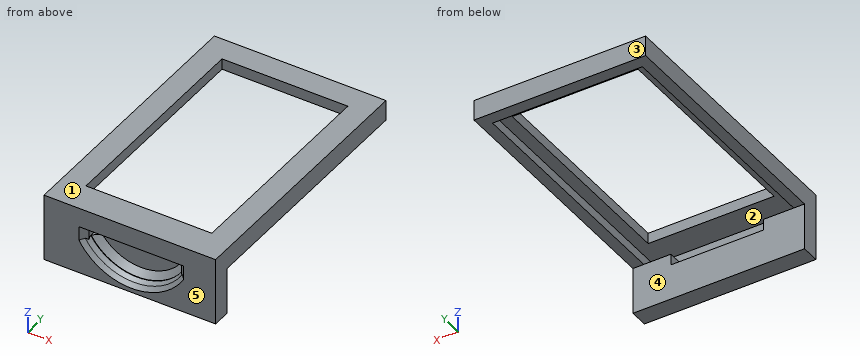
Autodesk Fusion 360 part; units mm, degrees
sketch "Sketch1" plane through (0, 0, 0) normal (0, 0, 1) x (1, 0, 0)
  line L0 (0, 0) -> (24.5, 0)
  line L1 (24.5, 0) -> (24.5, 42)
  line L2 (24.5, 42) -> (0, 42)
  line L3 (0, 42) -> (0, 0)
  line L4 (5, 39.4) -> (20, 39.4)
  line L5 (20, 39.4) -> (20, 24.4)
  line L6 (20, 24.4) -> (5, 24.4)
  line L7 (5, 24.4) -> (5, 39.4)
  dimension "d1" = 24.5
  dimension "d2" = 42
  dimension "d3" = 15
  dimension "d4" = 15
  dimension "d5" = 5
  dimension "d6" = 2.6
extrude "Extrude1" add sketch "Sketch1" along normal blind 1.2 contours L0 L1 L2 L3 | L4 L5 L6 L7 makes body 1
extrude "Extrude2" add sketch "Sketch1" against normal blind 1.85 contours L4 L5 L6 L7 bodies 1
sketch "Sketch2" plane through (0, 42, 0) normal (0, 1, 0) x (-1, 0, 0)
  line L0 (-24.5, 0) -> (0, 0)
  line L1 (0, 0) -> (0, 1.2)
  line L2 (0, 1.2) -> (-24.5, 1.2)
  line L3 (-24.5, 1.2) -> (-24.5, 0)
  line L4 (-26.5, 3.2) -> (2, 3.2)
  line L5 (2, 3.2) -> (2, -8)
  line L6 (2, -8) -> (-26.5, -8)
  line L7 (-26.5, -8) -> (-26.5, 3.2)
  line L8 (-20, 0) -> (-5, 0)
  line L9 (-5, 0) -> (-5, -1.85)
  line L10 (-5, -1.85) -> (-20, -1.85)
  line L11 (-20, -1.85) -> (-20, 0)
  line L12 (-20.2, 0.2) -> (-4.8, 0.2)
  line L13 (-4.8, 0.2) -> (-4.8, -2.05)
  line L14 (-4.8, -2.05) -> (-20.2, -2.05)
  line L15 (-20.2, -2.05) -> (-20.2, 0.2)
  line L16 (-24.7, 1.4) -> (0.2, 1.4)
  line L17 (0.2, 1.4) -> (0.2, -0.2)
  line L18 (0.2, -0.2) -> (-24.7, -0.2)
  line L19 (-24.7, -0.2) -> (-24.7, 1.4)
  arc A0 (-20.2, -2.05) -> (-4.8, -2.05) centre (-12.5, 2.7935) ccw
  line L20 (-26.5, 1.4) -> (2, 1.4)
  line L21 (2, 1.4) -> (2, 3.2)
  line L22 (2, 3.2) -> (-26.5, 3.2)
  line L23 (-26.5, 3.2) -> (-26.5, 1.4)
  line L24 (0.2, -0.2) -> (2, -0.2)
  line L25 (2, -0.2) -> (2, 1.4)
  line L26 (2, 1.4) -> (0.2, 1.4)
  line L27 (0.2, 1.4) -> (0.2, -0.2)
  line L28 (-24.7, -0.2) -> (-26.5, -0.2)
  line L29 (-26.5, -0.2) -> (-26.5, 1.4)
  line L30 (-26.5, 1.4) -> (-24.7, 1.4)
  line L31 (-24.7, 1.4) -> (-24.7, -0.2)
  dimension "d11" = 2
  dimension "d12" = 8
  dimension "d13" = 2
  dimension "d14" = 2
  dimension "d15" = 0.2
  dimension "d16" = 0.2
  dimension "d17" = 0.2
  dimension "d18" = 0.2
  dimension "d19" = 0.2
  dimension "d20" = 0.2
  dimension "d21" = 0.2
  dimension "d22" = 0.2
  dimension "d27" = 9.0967
  dimension "d33" = 0.2
extrude "Extrude3" add sketch "Sketch2" along normal blind 3 separate body contours L5 L6 L7 L13 L15 L18 A0 L24 L28 | L14 A0 | L7 L19 L20 L28 L29 L30 L31 | L5 L17 L20 L24 L25 L26 L27 | L4 L5 L7 L16 L20 L21 L22 L23 L26 L30 makes body 2
extrude "Extrude4" add sketch "Sketch2" along normal blind 0.4 contours L0 L8 L12 L13 L15 | L0 L1 L2 L3 L13 L15 L16 L17 L18 L19 L20 L27 L31 | L0 L1 L2 L3 L12 L13 L15 bodies 2
extrude "Extrude5" cut sketch "Sketch2" along normal blind 2.6 contours L14 A0 bodies 2
chamfer "Chamfer1" distance 1 angle 45 1 edges at (12.5, 44.6, -6.3032) on bodies 2
chamfer "Chamfer2" distance 1 angle 45 3 edges at (12.5, 42, -6.3032) (20.2, 42, -1.025) (4.8, 42, -1.025) on bodies 2
chamfer "Chamfer3" distance 0.5 angle 45 1 edges at (12.5, 43, -6.3032) on bodies 2
extrude "Extrude6" add sketch "Sketch2" along normal blind 44.6 contours L7 L19 L20 L28 L29 L30 L31 | L5 L17 L20 L24 L25 L26 L27 | L4 L5 L7 L16 L20 L21 L22 L23 L26 L30 bodies 2
sketch "Sketch3" plane through (0, 0, 1.4) normal (0, 0, -1) x (1, 0, 0)
  line L0 (24.7, -42.4) -> (-0.2, -42.4)
  line L1 (-0.2, -42.4) -> (-0.2, -86.6)
  line L2 (-0.2, -86.6) -> (24.7, -86.6)
  line L3 (24.7, -86.6) -> (24.7, -42.4)
  line L4 (-0.2, -86.6) -> (24.7, -86.6)
  line L5 (24.7, -86.6) -> (24.7, -84.6)
  line L6 (24.7, -84.6) -> (-0.2, -84.6)
  line L7 (-0.2, -84.6) -> (-0.2, -86.6)
  line L8 (1.8, -47) -> (22.7, -47)
  line L9 (22.7, -47) -> (22.7, -82.6)
  line L10 (22.7, -82.6) -> (1.8, -82.6)
  line L11 (1.8, -82.6) -> (1.8, -47)
  line L12 (26.5, -45) -> (-2, -45)
  dimension "d36" = 2
  dimension "d37" = 2
  dimension "d38" = 2
  dimension "d39" = 2
  dimension "d40" = 2
extrude "Extrude7" add sketch "Sketch3" along normal blind 1.6 contours L1 L2 L3 L4 L5 L6 L7 bodies 2
extrude "Extrude8" cut sketch "Sketch3" against normal blind 10 contours L8 L9 L10 L11 bodies 2
hidden bodies 1
equation "d34 = 42 mm + 0.6 mm + 2 mm"
Verification items for the finished model (mm, model axes). Face numbers are marked on the shaded views. A direction names the side the tool comes from. Give positions to 0.01 mm unless a question says otherwise; leave off trailing zeros. Loops run counter-clockwise (first coordinate to the right, second up) from the corner with the lowest first, then second, coordinate; pieces in that order, holes last.
1) Set-up check for the marked faces 4 and 5: record each of +Z, -Z, +X, -X, +Y, -Y from which the full face is reachable in a straight line by a thin tool's end or side.
2) Draft check along Z on the marked faces 1, 2 and 3. Enter one of: pulls with the +Z half, pulls with the -Z half, needs draft (parallel to the pull), parting line crosses it, or undercut.
3) Sectioned sample at B-B, the plane y = 51.5. Enter the section's corners in (x, z).
4) Depth check by flat-ended pin: pin 1 Ø10 at (x, y) = (7.5, 69.5) entering from +Z; pin 2 Ø1.5 at (x, z) = (5.5, -3) entering from -Y; pin 3 Ø10 at (x, y) = (23.5, 67.5) entering from -Z. Enter the tip coordinate at first touch or a pass-through.
5) Sectioned sample at D-D, the plane y = 84. Enter the section's corners in (x, z).
6) Sectioned sample at C-C, the plane x = 1. Enter the section's corners in (y, z), then the cut area to 3 significant figures.
7) Thickness scan on line 1 along Y through (x, z) = (12, 0.25); line 2 along X through (y, z) = (56, 1.5); line 3 along Y through (x, z) = (3, 2.5). Record the ranges inside material, lowest first.
8) Sectioned sample at A-A, the plane z = -1.5. Enter the section's corners in (x, y).
Answers:
1. face 4: -Z, +X, -X, +Y
1. face 5: +Z, -Z, +X, -X, -Y
2. face 1: pulls with the +Z half
2. face 2: undercut
2. face 3: needs draft
3. outline: (-2, -0.2) - (-0.2, -0.2) - (-0.2, 1.4) - (1.8, 1.4) - (1.8, 3.2) - (-2, 3.2) - close; (22.7, 1.4) - (24.7, 1.4) - (24.7, -0.2) - (26.5, -0.2) - (26.5, 3.2) - (22.7, 3.2) - close
4. pin 1: passes through
4. pin 2: stops at y = 42.26
4. pin 3: stops at z = -0.2
5. outline: (-2, -0.2) - (-0.2, -0.2) - (-0.2, 1.4) - (24.7, 1.4) - (24.7, -0.2) - (26.5, -0.2) - (26.5, 3.2) - (-2, 3.2) - close
6. outline: (42, -8) - (45, -8) - (45, -0.2) - (42.4, -0.2) - (42.4, 1.4) - (84.6, 1.4) - (84.6, -0.2) - (86.6, -0.2) - (86.6, 3.2) - (42, 3.2) - close
6. area: 108 mm2
7. line 1: y = 42 to 42.4, 84.6 to 86.6
7. line 2: x = -2 to 1.8, 22.7 to 26.5
7. line 3: y = 42 to 47, 82.6 to 86.6
8. outline: (-2, 42) - (3.8, 42) - (4.8, 43) - (4.8, 45) - (-2, 45) - close; (20.2, 43) - (21.2, 42) - (26.5, 42) - (26.5, 45) - (20.2, 45) - close
